Here's how the part is built. I have some questions about the finished solid (model axes, mm). Face numbers are marked on the shaded views. A direction names the side the tool comes from. Round coordinates to 2 decimals unless told otherwise and drop trailing zeros. Order: outer loops, then holes, each group sorted by start corner. A loop starts at its lowest first (then second) coordinate and runs counter-clockwise, first axis right, second up. Notation, with made-up numbers: (-29, 86) - (17, 86) arc R21 cw to (17, 117) - close; hole circle Ø1 at (84, -30). An arc over 180 degrees is marked (long way). One line per item, written item: value.
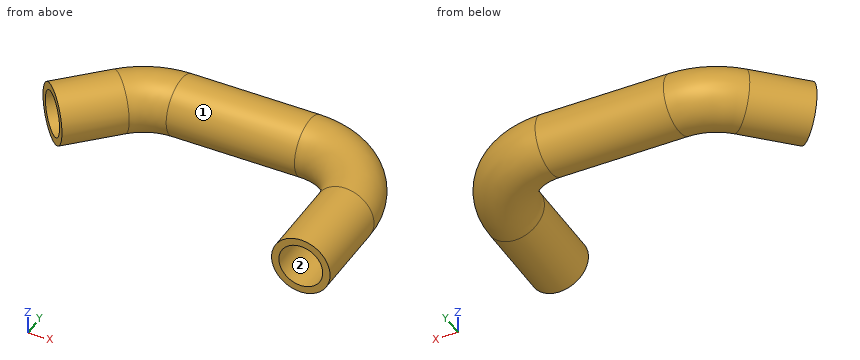
from build123d import *

# Parameters (mm, degrees)
F0_R   = 2.54
F0_R_2 = 1.905


with BuildPart() as f2:
    # F2: sweep along a path in F1
    with BuildLine(Plane.XY) as f2_path:
        Line((0, 0), (0, 7.3384581298))
        ThreePointArc((0, 7.3384581298), (-1.8598719395, 11.8285861903), (-6.35, 13.6884581298))
        Line((-6.35, 13.6884581298), (-12.5316856429, 13.6884581298))
        Line((-12.5316856429, 13.6884581298), (-17.4858820379, 13.6884581298))
        ThreePointArc((-17.4858820379, 13.6884581298), (-19.8729520403, 13.2227080228), (-21.9098557091, 11.8937799577))
        Line((-21.9098557091, 11.8937799577), (-25.7876180112, 8.12782906))
    # F0 (on Front) → F2 (sweep)
    with BuildSketch(Plane.XZ):
        Circle(F0_R)
        Circle(F0_R_2, mode=Mode.SUBTRACT)
    sweep(path=f2_path.line)


solid = f2.part
Q1. If we section it at B-B, the plane y = 1.5: Please give me the cut outline in (x, z) (3 decimals), then the cut area to 3 significant figures.
Results list:
outline: circle Ø5.08 at (0, 0); hole circle Ø3.81 at (0, 0)
area: 8.87 mm²
Q2. Which directions (+Z, -Z, +X, -X, +Y, -Y) give clear straight access to the entire face, cutting with the end or side of a thin tool? Please do the marked faces 1 and 2.
Results list:
face 1: none
face 2: -Y
Q3. If we section it at A-A, the plane z = 1.55: Please give me the cut outline in (x, y).
Results list:
outline: (-27.19, 9.57) - (-26.56, 8.92) - (-22.68, 12.69) arc R7.46 cw to (-17.49, 14.8) - (-6.35, 14.8) arc R7.46 cw to (1.11, 7.34) - (1.11, 0) - (2.01, 0) - (2.01, 7.34) arc R8.36 ccw to (-6.35, 15.7) - (-17.49, 15.7) arc R8.36 ccw to (-23.31, 13.34) - close; (-25.02, 7.33) - (-24.39, 6.68) - (-20.51, 10.45) arc R4.34 cw to (-17.49, 11.68) - (-6.35, 11.68) arc R4.34 cw to (-2.01, 7.34) - (-2.01, 0) - (-1.11, 0) - (-1.11, 7.34) arc R5.24 ccw to (-6.35, 12.58) - (-17.49, 12.58) arc R5.24 ccw to (-21.14, 11.1) - close
Q4. If I drill on line 1 along Y through (x, z) = (-11, 0); line 2 along Z through (x, y) = (0, 4.75) (3 decimals), over which ranges is the centre line in solid material (lowest first)?
Results list:
line 1: 11.15 to 11.78, 15.59 to 16.23
line 2: -2.54 to -1.905, 1.905 to 2.54
Q5. Will these pins go through, and if not, where does the flat tip stop? pin 1 (2 mm diameter, centred on x = -4, z = 1.5, fed in from +Y); pin 2 (1 mm diameter, centred on y = 8.5, z = 0.5, fed in from -X); pin 3 (3 mm diameter, centred on x = -8, z = -1, fed in from -Y).
Results list:
pin 1: y = 15.95
pin 2: x = -23.34
pin 3: y = 11.15
Q6. If we section it at D-D, the plane x = -16.5: Please give me the cut outline in (y, z) (3 decimals).
Results list:
outline: circle Ø5.08 at (13.688, 0); hole circle Ø3.81 at (13.688, 0)
Q7. If we section it at C-C, the plane z = -0.95: Please give me the cut outline in (x, y).
Results list:
outline: (-27.43, 9.82) - (-26.94, 9.31) - (-23.06, 13.08) arc R8 cw to (-17.49, 15.34) - (-6.35, 15.34) arc R8 cw to (1.65, 7.34) - (1.65, 0) - (2.36, 0) - (2.36, 7.34) arc R8.71 ccw to (-6.35, 16.04) - (-17.49, 16.04) arc R8.71 ccw to (-23.55, 13.58) - close; (-24.64, 6.94) - (-24.15, 6.44) - (-20.27, 10.2) arc R3.99 cw to (-17.49, 11.33) - (-6.35, 11.33) arc R3.99 cw to (-2.36, 7.34) - (-2.36, 0) - (-1.65, 0) - (-1.65, 7.34) arc R4.7 ccw to (-6.35, 12.04) - (-17.49, 12.04) arc R4.7 ccw to (-20.76, 10.71) - close
